from build123d import *

# Parameters (mm, degrees)
BOSS_EXTRUDE1_DEPTH = 375
FILLET1_R           = 2.032
FILLET2_R           = 1.27
SKETCH5_W           = 12.048677603
SKETCH5_H           = 11.996966541
SKETCH5_R           = 1.809887194
SKETCH5_R_2         = 1.778
SKETCH5_R_3         = 1.784780941
CUT_EXTRUDE3_DEPTH  = 376.626052464
SCALE1_SCALE        = 0.8


with BuildPart() as part:
    # Sketch2 → Boss-Extrude1 (new body)
    with BuildSketch(Plane(origin=(0, 0, 0), x_dir=(1, 0, 0), z_dir=(0, 1, 0))):
        Polygon((-11.631944508, 4.856112595), (-11.631944508, -8.62647921), (-15.607851567, -2.645315933), (-16.258611825, -14.593573265), (-4.310354494, -13.942813006), (-10.340832945, -9.861953178), (3.339587632, -9.861953178), (-2.854456203, -13.936328227), (9.141388175, -14.593573265), (8.484143137, -2.597728887), (4.461618468, -8.47589662), (4.461618468, 4.675168062), (8.490627916, 0), (9.141388175, 10.806426735), (-1.66503856, 10.155666477), (3.011955341, 6.231609797), (-10.257604353, 6.231609797), (-4.292081103, 10.155666477), (-16.258611825, 10.806426735), (-15.607851567, -1.160103987), align=None)
    extrude(amount=BOSS_EXTRUDE1_DEPTH)

    # Fillet1
    fillet1_edges = [part.edges().sort_by_distance(p)[0] for p in [
        (9.141388175, 187.5, 14.593573265),
        (-16.258611825, 187.5, 14.593573265),
        (-16.258611825, 187.5, -10.806426735),
        (9.141388175, 187.5, -10.806426735),
    ]]
    fillet(fillet1_edges, radius=FILLET1_R)

    # Fillet2
    fillet2_edges = [part.edges().sort_by_distance(p)[0] for p in [
        (8.490627916, 187.5, 0),
        (8.484143137, 187.5, 2.597728887),
        (-2.854456203, 187.5, 13.936328227),
        (-4.310354494, 187.5, 13.942813006),
        (-15.607851567, 187.5, 2.645315933),
        (-15.607851567, 187.5, 1.160103987),
        (-4.292081103, 187.5, -10.155666477),
        (-1.66503856, 187.5, -10.155666477),
    ]]
    fillet(fillet2_edges, radius=FILLET2_R)

    # Sketch5 → Cut-Extrude3 (cut, through all)
    with BuildSketch(Plane(origin=(0, 375, 0), x_dir=(1, 0, 0), z_dir=(0, 1, 0))):
        with Locations((-3.593458736, -1.901154881)):
            Rectangle(SKETCH5_W, SKETCH5_H)
        with Locations(Location((6.050654454, -11.415990413, 0), (0, 0, 270))):
            Circle(SKETCH5_R)
        with Locations(Location((-13.030727673, -11.545268069, 0), (0, 0, 270))):
            Circle(SKETCH5_R_2)
        with Locations(Location((-13.108294267, 7.613680652, 0), (0, 0, 270))):
            Circle(SKETCH5_R_2)
        with Locations(Location((5.921376797, 7.665391714, 0), (0, 0, 270))):
            Circle(SKETCH5_R_3)
    extrude(amount=-CUT_EXTRUDE3_DEPTH, mode=Mode.SUBTRACT)


with BuildPart() as part_1:
    # Scale1: scaled about (-3.644090286, 187.5, 1.930683285)
    add(part.part.scale(SCALE1_SCALE).moved(Location((-0.728818057, 37.5, 0.386136657))))


solid = part_1.part
Part model, mm, in its own coordinate system. A direction names the side the tool comes from. Coordinates: 2 decimals unless noted, no trailing zeros. Write each question's results on one line, items separated by ' | '. Start each with the question number.
Q1. Which spindle directions (+Z, -Z, +X, -X, +Y, -Y) get a long thin tool onto all of the face, cutting with end or side? Do faces 4 (the flat face through (-9.592, 185.4, 11.835)), 5 (the flat face through (-4, 190, -2.892)), 6 (the flat face through (-13.51, 185.4, -4.14)), 7 (the flat face through (-9.55, 185.4, -8.03)), 8 (the flat face through (-9, 37.5, 3)). Say none if no direction does.
Q2. Probe line 1 along Z through (x, y) = (-5.75, 262); line 2 along X through (y, z) = (263.5, 8.75); line 3 along X through (y, z) = (119, 5.25). List the from-to ranges inside material, lowest first.
Q3. Two-plate mould, pull along X, no slides. Class faces 1 (the flat face through (-9, 337.5, 3)), 2 (the flat face through (2.84, 185, 2)), 3 (the flat face through (6.355, 185.4, 7.884)): +X half, -X half, draft (parallel to the pull), parting line (faces both ways), or undercut.
Q4. Slice it at A-A on y = 78. Give the number of separate pieces and of enclosed holes in the cut face, and give its area (3 significant figures).
Q5. Drop flat-ended pins along their axis: pin 1 Ø1.5 at (y, z) = (92, 3) entering from +X; pin 2 Ø8.5 at (x, y) = (-3, 209) entering from -Z; pin 3 Ø1 at (x, y) = (1, 230) entering from -Z. Give the stop position or say it passes through.
Answer:
1) face 4: +Z, +Y, -Y | face 5: +Y, -Y | face 6: -X, +Y, -Y | face 7: -Z, +Y, -Y | face 8: +Z, -Z, +X, -X, -Y
2) line 1: z = -4.6 to -2.89, 6.71 to 8.28 | line 2: x = -13.56 to -12.28, -10.03 to -8.3, 1.22 to 2.88, 5.34 to 6.4 | line 3: x = -13.32 to -11.39, -10.03 to -8.42, 1.22 to 2.84, 4.15 to 6.19
3) face 1: draft | face 2: undercut | face 3: +X half
4) separate pieces: 1 | enclosed holes: 5 | area: 176 mm2
5) pin 1: stops at x = 2.84 | pin 2: stops at z = -7.94 | pin 3: stops at z = -7.95
